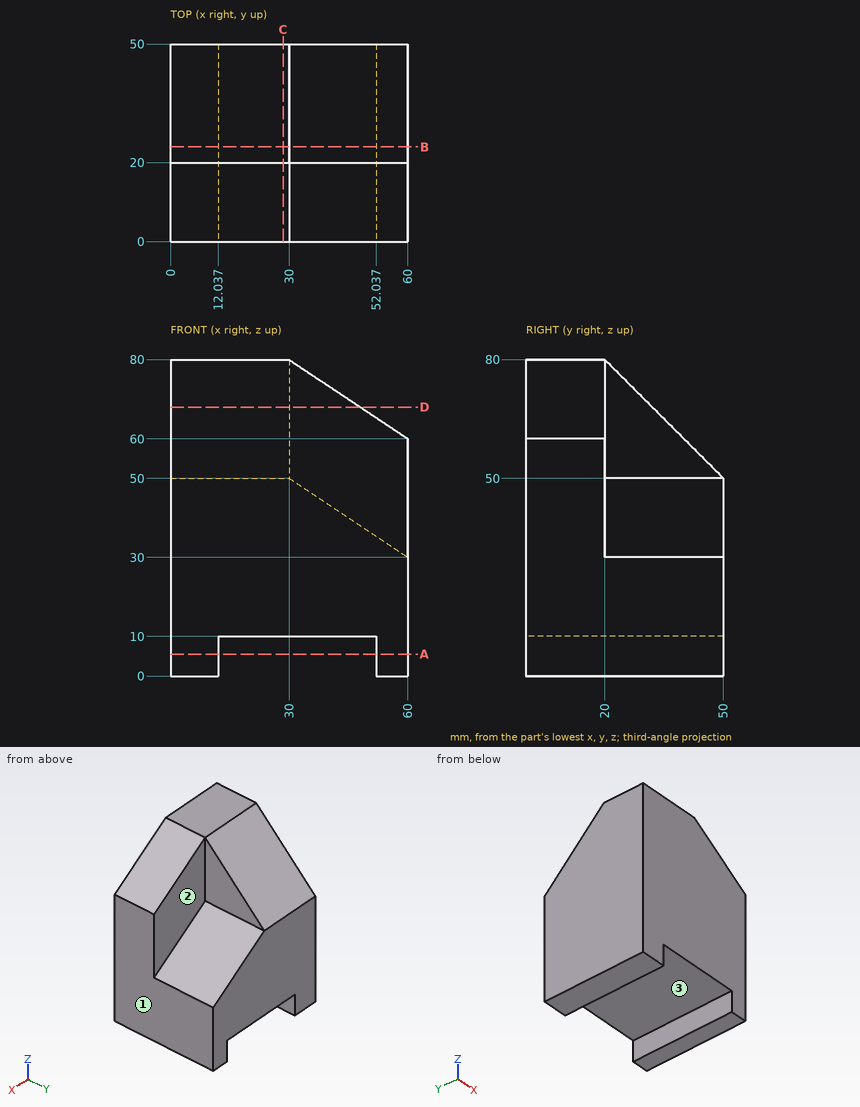
Source: three-view drawing plus pictorial views. Frame: mm from the lowest corner of the part. A direction names the side the tool comes from. Round coordinates to 2 decimals unless told otherwise and drop trailing zeros. Order: outer loops, then holes, each group sorted by start corner. A loop starts at its lowest first (then second) coordinate and runs counter-clockwise, first axis right, second up. Notation, with made-up numbers: (-21.5, 20) - (-0.5, 20) arc R18 cw to (-0.5, 43) - close; hole circle Ø8 at (30, 71). An arc over 180 degrees is marked (long way). Write each question's results on one line, items separated by ' | '.
Item 1: Material intervals for line 1 along X through (y, z) = (35.5, 8); line 2 along Z through (x, y) = (18, 15); line 3 along X through (y, z) = (42, 50.5), sorted ascending. Write a range as [from, to].
Completed:
line 1: [0, 12.04], [52.04, 60] | line 2: [10, 80] | line 3: [0, 30]
Item 2: Section A-A, the plane z = 5.5. Return the cut outline in (x, y).
Completed:
outline: (0, 0) - (12.04, 0) - (12.04, 50) - (0, 50) - close; (52.04, 0) - (60, 0) - (60, 50) - (52.04, 50) - close
Item 3: Section D-D, the plane z = 68. Return the cut outline in (x, y), and give its area (3 significant figures).
Completed:
outline: (0, 0) - (48, 0) - (48, 20) - (30, 20) - (30, 32) - (0, 32) - close | area: 1,320 mm^2
Item 4: Reachability of the marked faces 1, 2 and 3 from +Z, -Z, +X, -X, +Y, -Y: full face, straight path, thin tool, end or side. Return the list, or none.
Completed:
face 1: +Z, -Z, +X, +Y, -Y | face 2: +Z, +X, +Y | face 3: -Z, +Y, -Y
Item 5: Section B-B, the plane y = 24. Return the cut outline in (x, z), and give its area (3 significant figures).
Completed:
outline: (0, 0) - (12.04, 0) - (12.04, 10) - (52.04, 10) - (52.04, 0) - (60, 0) - (60, 30) - (30, 50) - (30, 76) - (0, 76) - close | area: 3,080 mm^2
Item 6: First-contact query: pin 1 Ø12 at (y, z) = (27, 69.5) entering from +X; pin 2 Ø4 at (x, y) = (15, 24) entering from +Z; pin 3 Ø2 at (x, y) = (16.5, 14) entering from -Z. Flat tips, straight axial feed; report the tip coordinate or a pass-through.
Completed:
pin 1: x = 30 | pin 2: z = 78 | pin 3: z = 10
Item 7: Section C-C, the plane x = 28.5. Return the cut outline in (y, z), and give its area (3 significant figures).
Completed:
outline: (0, 10) - (50, 10) - (50, 50) - (20, 80) - (0, 80) - close | area: 3,050 mm^2
